from build123d import *

# Parameters (mm, degrees)
BOSS_EXTRUDE1_DEPTH = 45
SKETCH2_W           = 31
SKETCH2_H           = 37
BOSS_EXTRUDE3_START = -45
BOSS_EXTRUDE3_DEPTH = 45
SKETCH4_R           = 5.05
CUT_EXTRUDE1_DEPTH  = 12
SKETCH5_W           = 5
SKETCH5_H           = 35
CUT_EXTRUDE2_DEPTH  = 67.895440801
BOSS_EXTRUDE5_DEPTH = 37
BOSS_EXTRUDE6_START = 5
SKETCH7_W           = 17.5
SKETCH7_H           = 7.441015215
BOSS_EXTRUDE6_DEPTH = 5
SKETCH9_W           = 15
SKETCH9_H           = 55
SKETCH9_W_2         = 10
BOSS_EXTRUDE7_DEPTH = 3
SKETCH12_R          = 1.55
CUT_EXTRUDE5_DEPTH  = 5
SKETCH13_W          = 7
SKETCH13_H          = 4
CUT_EXTRUDE6_DEPTH  = 90.162772501
CUT_EXTRUDE7_DEPTH  = 74.993242935


with BuildPart() as part:
    # Sketch1 → Boss-Extrude1 (new body)
    with BuildSketch(Plane.XY):
        with BuildLine():
            Line((35, 0), (-35, 0))
            ThreePointArc((-35, 0), (0, -35), (35, 0))
        make_face()
    extrude(amount=BOSS_EXTRUDE1_DEPTH)

    # Sketch2 → Cut-Revolve1 (revolve, cut)
    with BuildSketch(Plane(origin=(0, 0, 0), x_dir=(1, 0, 0), z_dir=(0, 1, 0))):
        with Locations((-15.5, -22.5)):
            Rectangle(SKETCH2_W, SKETCH2_H)
    revolve(axis=Axis((0, 0, 0), (0, 0, 1)), mode=Mode.SUBTRACT)

    # Sketch3 → Boss-Extrude3 (add)
    with BuildSketch(Plane.XY.offset(45).offset(BOSS_EXTRUDE3_START)):
        with BuildLine():
            Line((-17.5, -35), (-17.5, -30.310889132))
            ThreePointArc((-17.5, -30.310889132), (-30.310889132, -17.5), (-35, 0))
            Line((-35, 0), (-35, -35))
            Line((-35, -35), (-17.5, -35))
        make_face()
        with BuildLine():
            ThreePointArc((0, -35), (-9.058666579, -33.80740392), (-17.5, -30.310889132))
            Line((-17.5, -30.310889132), (-17.5, -35))
            Line((-17.5, -35), (0, -35))
        make_face()
        with BuildLine():
            Line((-17.5, -30.310889132), (-17.5, 0))
            Line((-17.5, 0), (-35, 0))
            ThreePointArc((-35, 0), (-30.310889132, -17.5), (-17.5, -30.310889132))
        make_face()
    extrude(amount=BOSS_EXTRUDE3_DEPTH)

    # Sketch4 → Cut-Extrude1 (cut)
    with BuildSketch(Plane.ZY.offset(35)):
        with Locations((10, -17.5)):
            Circle(SKETCH4_R)
        with Locations(Location((35, -17.5, 0), (0, 0, 180))):
            Circle(SKETCH4_R)
    extrude(amount=-CUT_EXTRUDE1_DEPTH, mode=Mode.SUBTRACT)

    # Sketch5 → Cut-Extrude2 (cut, through all)
    with BuildSketch(Plane(origin=(0, 0, 0), x_dir=(-1, 0, 0), z_dir=(0, 0, -1))):
        with Locations((32.5, -17.5)):
            Rectangle(SKETCH5_W, SKETCH5_H)
    extrude(amount=-CUT_EXTRUDE2_DEPTH, mode=Mode.SUBTRACT)

    # Sketch6 → Boss-Extrude5 (add)
    with BuildSketch(Plane(origin=(0, 0, 41), x_dir=(-1, 0, 0), z_dir=(0, 0, -1))):
        with BuildLine():
            ThreePointArc((-31, 0), (-25.966324345, -16.933694222), (-12.5, -28.368115905))
            Line((-12.5, -28.368115905), (-12.5, 0))
            Line((-12.5, 0), (-31, 0))
        make_face()
        with BuildLine():
            Line((12.5, 0), (12.5, -28.368115905))
            ThreePointArc((12.5, -28.368115905), (15.064267175, -27.093686617), (17.5, -25.588083164))
            Line((17.5, -25.588083164), (17.5, 0))
            Line((17.5, 0), (12.5, 0))
        make_face()
    extrude(amount=BOSS_EXTRUDE5_DEPTH)

    # Sketch7 → Boss-Extrude6 (add)
    with BuildSketch(Plane(origin=(0, 0, 0), x_dir=(-1, 0, 0), z_dir=(0, 0, -1)).offset(BOSS_EXTRUDE6_START)):
        with BuildLine():
            Line((-12.5, 0), (-35, 0))
            ThreePointArc((-35, 0), (-34.799393274, -3.741955075), (-34.199872698, -7.441015215))
            Line((-34.199872698, -7.441015215), (-12.5, -7.441015215))
            Line((-12.5, -7.441015215), (-12.5, 0))
        make_face()
        with Locations((21.25, -3.720507608)):
            Rectangle(SKETCH7_W, SKETCH7_H)
    boss_extrude6 = extrude(amount=-BOSS_EXTRUDE6_DEPTH)

    # Mirror1: Boss-Extrude6 across plane
    add(boss_extrude6.mirror(Plane(origin=(0, 0, 22.5), x_dir=(1, 0, 0), z_dir=(0, 0, -1))))

    # Sketch9 → Boss-Extrude7 (add)
    with BuildSketch(Plane(origin=(0, 0, 0), x_dir=(1, 0, 0), z_dir=(0, 1, 0))):
        with Locations((27.5, -22.5)):
            Rectangle(SKETCH9_W, SKETCH9_H)
        with Locations((-25, -22.5)):
            Rectangle(SKETCH9_W_2, SKETCH9_H)
    extrude(amount=BOSS_EXTRUDE7_DEPTH)

    # Sketch12 → Cut-Extrude5 (cut)
    with BuildSketch(Plane(origin=(0, 3, 0), x_dir=(1, 0, 0), z_dir=(0, 1, 0))):
        with Locations(Location((26, 1.5, 0), (0, 0, 270))):
            Circle(SKETCH12_R)
        with Locations(Location((26, -10.5, 0), (0, 0, 270))):
            Circle(SKETCH12_R)
        with Locations(Location((26, -34.5, 0), (0, 0, 90))):
            Circle(SKETCH12_R)
        with Locations(Location((26, -46.5, 0), (0, 0, 90))):
            Circle(SKETCH12_R)
        with Locations(Location((-26, 1.5, 0), (0, 0, 90))):
            Circle(SKETCH12_R)
        with Locations(Location((-26, -10.5, 0), (0, 0, 90))):
            Circle(SKETCH12_R)
        with Locations(Location((-26, -34.5, 0), (0, 0, 270))):
            Circle(SKETCH12_R)
        with Locations(Location((-26, -46.5, 0), (0, 0, 270))):
            Circle(SKETCH12_R)
    extrude(amount=-CUT_EXTRUDE5_DEPTH, mode=Mode.SUBTRACT)

    # Sketch13 → Cut-Extrude6 (cut, through all)
    with BuildSketch(Plane(origin=(35, 0, 0), x_dir=(0, 0, -1), z_dir=(1, 0, 0))):
        with Locations((-46.5, -2)):
            Rectangle(SKETCH13_W, SKETCH13_H)
        with Locations((-34.5, -2)):
            Rectangle(SKETCH13_W, SKETCH13_H)
        with Locations((-10.5, -2)):
            Rectangle(SKETCH13_W, SKETCH13_H)
        with Locations((1.5, -2)):
            Rectangle(SKETCH13_W, SKETCH13_H)
    extrude(amount=-CUT_EXTRUDE6_DEPTH, mode=Mode.SUBTRACT)

    # Sketch14 → Cut-Extrude7 (cut, through all)
    with BuildSketch(Plane.XY.offset(50)):
        Polygon((-17.094187338, 0), (35.300582727, 0), (35.300582727, -35.487417881), (-30, -35.487417881), (-30, 0), (-30, 9.051842105), (-17.094187338, 9.051842105), align=None)
    extrude(amount=-CUT_EXTRUDE7_DEPTH, mode=Mode.SUBTRACT)


solid = part.part
CAD build for the part. Positions are in the model's coordinates, mm. Round coordinates to 2 decimals unless told otherwise and drop trailing zeros. Order: outer loops, then holes, each group sorted by start corner. A loop starts at its lowest first (then second) coordinate and runs counter-clockwise, first axis right, second up. Notation, with made-up numbers: (16, -4.75) -> (64, -4.75) arc R22 cw to (64, 32.25) -> close; hole circle Ø6 at (13.25, 83.5). An arc over 180 degrees is marked (long way). Write each question's results on one line, items separated by ' | '.
1. Pull direction X, two halves, no side cores. Call faces 1 (the face through (20, 1, 23)), 2 (the face through (27, 1, -5)), 3 (the face through (25.534, 1.521, 45.022)): pulls with the +X half, pulls with the -X half, needs draft (parallel to the pull), parting line crosses it, or undercut.
Findings below:
face 1: pulls with the -X half | face 2: needs draft | face 3: undercut
2. Cut at B-B (z = -1.5). Give the cut face in (x, y), plus the area to 3 significant figures.
Findings below:
outline: (20, 0) -> (24.45, 0) -> (24.45, 3) -> (20, 3) -> close; (27.55, 0) -> (35, 0) -> (35, 3) -> (27.55, 3) -> close | area: 35.7 mm²
3. Cut at A-A (y = 2.35). Give the cut face in (x, z).
Findings below:
outline: (20, -5) -> (35, -5) -> (35, 50) -> (20, 50) -> close; hole circle Ø3.1 at (26, -1.5); hole circle Ø3.1 at (26, 10.5); hole circle Ø3.1 at (26, 34.5); hole circle Ø3.1 at (26, 46.5)
4. Flat gauge pin, fed straight in: P1, Ø3, axis at x = 26, z = 34.5, coming from the -Y side. Where does the tip first touch, or does it go through?
Findings below:
P1: passes through
5. Wall check: line 1 along X through (y, z) = (1.9, 10.5). Give the ranges that are in metal, low to high. Write a range as [from, to].
Findings below:
line 1: x = [20, 24.45], [27.55, 35]
6. Cut at C-C (x = 26). Give the cut face in (y, z), plus the area to 3 significant figures.
Findings below:
outline: (0, -5) -> (3, -5) -> (3, -3.05) -> (0, -3.05) -> close; (0, 0.05) -> (3, 0.05) -> (3, 8.95) -> (0, 8.95) -> close; (0, 12.05) -> (3, 12.05) -> (3, 32.95) -> (0, 32.95) -> close; (0, 36.05) -> (3, 36.05) -> (3, 44.95) -> (0, 44.95) -> close; (0, 48.05) -> (3, 48.05) -> (3, 50) -> (0, 50) -> close | area: 128 mm²
